```python
from build123d import *

# Parameters (mm, degrees)
SKETCH013_W     = 80
SKETCH013_H     = 28
PAD007_DEPTH    = 3.6
SKETCH014_R     = 3
SKETCH014_R_2   = 1.1
PAD008_DEPTH    = 2
SKETCH016_R     = 1
POCKET003_DEPTH = 5


with BuildPart() as part:
    # Sketch013 → Pad007 (new body)
    with BuildSketch(Plane.XY):
        with BuildLine():
            Line((0, -3), (85, -3))
            ThreePointArc((85, -3), (87.12132, -2.12132), (88, 0))
            Line((88, 0), (88, 28))
            ThreePointArc((88, 28), (87.12132, 30.12132), (85, 31))
            Line((85, 31), (0, 31))
            ThreePointArc((0, 31), (-2.12132, 30.12132), (-3, 28))
            Line((-3, 28), (-3, 0))
            ThreePointArc((-3, 0), (-2.12132, -2.12132), (0, -3))
        make_face()
        with Locations((42, 14)):
            Rectangle(SKETCH013_W, SKETCH013_H, mode=Mode.SUBTRACT)
    extrude(amount=PAD007_DEPTH)

    # Sketch014 → Pad008 (join)
    with BuildSketch(Plane.XY):
        with Locations((4.637, 20.614)):
            Circle(SKETCH014_R)
        with Locations((4.637, 20.614)):
            Circle(SKETCH014_R_2, mode=Mode.SUBTRACT)
        with Locations((54.675, 25.44)):
            Circle(SKETCH014_R)
        with Locations((54.675, 25.44)):
            Circle(SKETCH014_R_2, mode=Mode.SUBTRACT)
        with Locations((54.675, 2.58)):
            Circle(SKETCH014_R)
        with Locations((54.675, 2.58)):
            Circle(SKETCH014_R_2, mode=Mode.SUBTRACT)
    extrude(amount=PAD008_DEPTH)

    # Sketch016 → Pocket003 (cut)
    with BuildSketch(Plane.XY.offset(2)):
        with Locations((2, 28)):
            Circle(SKETCH016_R)
        with Locations((82, 28)):
            Circle(SKETCH016_R)
        with Locations((82, 0)):
            Circle(SKETCH016_R)
        with Locations((2, 0)):
            Circle(SKETCH016_R)
    extrude(amount=POCKET003_DEPTH, mode=Mode.SUBTRACT)


solid = part.part
```
CAD build for the part. Positions are in the model's coordinates, mm. A direction names the side the tool comes from. Coordinates: 2 decimals unless noted, no trailing zeros. Write each loop counter-clockwise with the first axis right and the second up, starting at its lowest first coordinate (ties: lowest second). Pieces come first, ordered by that corner, then holes. Notation, with made-up numbers: (21, 63.25) -> (71, 63.25) arc R21 cw to (71, 79.25) -> close; hole circle Ø6 at (67.25, 64). An arc over 180 degrees is marked (long way). Use CSV: the item, a comma, the result in double quotes. Start each with the question number.
Item 1: Two-plate mould, pull along X, no slides. Class faces 4 (the cylindrical face through (82.683, -0.73, 2.789)), 5 (the flat face through (42, -3, 2)), 6 (the flat face through (-3, 14, 2)), 7 (the flat face through (41, 0, 2)): +X half, -X half, draft (parallel to the pull), parting line (faces both ways), or undercut.
Item 2: Band-saw the part on B-B, the plane x = 70.5. Write the cut outline in (y, z).
Item 3: Band-saw the part on A-A, the plane y = 2.58. Write the cut outline in (x, z) (3 decimals), plus the area to 3 significant figures.
Item 4: Wall check: probe 1 along Y at (x, z) = (44.5, 2.5); probe 2 along Y at (x, z) = (6, 1.05); probe 3 along X at (y, z) = (17, 1.05). Give the ranges that are in metal, low to high.
Item 5: Band-saw the part on C-C, the plane y = 15. Write the cut outline in (x, z), plus the area to 3 significant figures.
Item 6: Drop a flat-ended pin along its axis: P1, Ø3.5, axis at x = 54.675, y = 25.44, coming from the +Z side. Give the stop position or say it passes through.
Item 7: Tool access for faces 1 (the flat face through (88, 14, 2)), 2 (the flat face through (82, 14, 2)), 3 (the flat face through (1.8, 28, 2)): list every direction of +Z, -Z, +X, -X, +Y, -Y with a clear straight run to the whole face (end or side of a thin tool).
Response values:
1,face 4,"undercut"
1,face 5,"draft"
1,face 6,"-X half"
1,face 7,"undercut"
2,outline,"(-3, 0) -> (0, 0) -> (0, 3.6) -> (-3, 3.6) -> close; (28, 0) -> (31, 0) -> (31, 3.6) -> (28, 3.6) -> close"
3,outline,"(-3, 0) -> (2, 0) -> (2, 3.6) -> (-3, 3.6) -> close; (51.675, 0) -> (53.575, 0) -> (53.575, 2) -> (51.675, 2) -> close; (55.775, 0) -> (57.675, 0) -> (57.675, 2) -> (55.775, 2) -> close; (82, 0) -> (88, 0) -> (88, 3.6) -> (82, 3.6) -> close"
3,area,"47.2 mm2"
4,probe 1,"y = -3 to 0, 28 to 31"
4,probe 2,"y = -3 to 0, 17.94 to 23.29, 28 to 31"
4,probe 3,"x = -3 to 2, 82 to 88"
5,outline,"(-3, 0) -> (2, 0) -> (2, 3.6) -> (-3, 3.6) -> close; (82, 0) -> (88, 0) -> (88, 3.6) -> (82, 3.6) -> close"
5,area,"39.6 mm2"
6,P1,"stops at z = 2"
7,face 1,"+Z, -Z, +X, +Y, -Y"
7,face 2,"+Z, -Z"
7,face 3,"+Z"
